Geometry check sheet. Reference: the model listing, model coordinates, mm. Face numbers are marked on the shaded views. A direction names the side the tool comes from. Give positions to 0.01 mm unless a question says otherwise; leave off trailing zeros. Loops run counter-clockwise (first coordinate to the right, second up) from the corner with the lowest first, then second, coordinate; pieces in that order, holes last. Notation, with made-up numbers: (-18.5, 22) -> (18.5, 22) arc R23 ccw to (18.5, 31) -> close; hole circle Ø6 at (32, 75). An arc over 180 degrees is marked (long way). Answer in a Markdown table with one row per item. Add a question column.
```python
from build123d import *

# Parameters (mm, degrees)
SKETCH1_R           = 43.5
BOSS_EXTRUDE1_DEPTH = 11.35
CHAMFER1_SIZE       = 2
SKETCH2_R           = 10.5


with BuildPart() as part:
    # Sketch1 → Boss-Extrude1 (new, symmetric)
    with BuildSketch(Plane.XY):
        Circle(SKETCH1_R)
        with BuildLine():
            Line((-5, 18.142135624), (5, 18.142135624))
            Line((5, 18.142135624), (5, 14.142135624))
            ThreePointArc((5, 14.142135624), (0, -15), (-5, 14.142135624))
            Line((-5, 14.142135624), (-5, 18.142135624))
        make_face(mode=Mode.SUBTRACT)
    extrude(amount=BOSS_EXTRUDE1_DEPTH, both=True)

    # Chamfer1
    chamfer1_edges = [part.edges().sort_by_distance(p)[0] for p in [
        (-43.5, 0, -11.35),
        (-43.5, 0, 11.35),
    ]]
    chamfer(chamfer1_edges, length=CHAMFER1_SIZE)

    # Sketch2 → Cut-Revolve1 (revolve, cut)
    with BuildSketch(Plane(origin=(0, 0, 0), x_dir=(0, 0, -1), z_dir=(1, 0, 0)), mode=Mode.PRIVATE) as cut_revolve1_sk:
        with Locations((0, -52)):
            Circle(SKETCH2_R)
    revolve(cut_revolve1_sk.sketch.rotate(Axis((0, 0, -83.533331893), (0, 0, 1)), 270), axis=Axis((0, 0, -83.533331893), (0, 0, 1)), mode=Mode.SUBTRACT)


solid = part.part
```
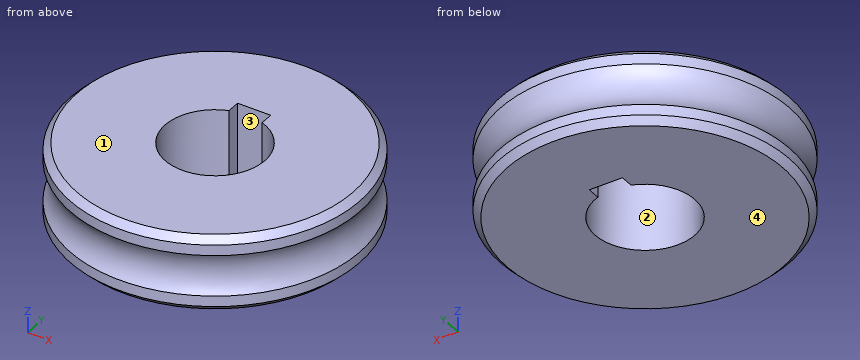
1. Sectioned sample at B-B (x = 0). Enter the section's corners in (y, z), plus the area to 3 significant figures.
2. Sectioned sample at C-C (z = 3.5). Enter the section's corners in (x, y).
3. Gauge pin test, flat ends, axial feed: pin 1 Ø3 at (y, z) = (16.5, 1.5) entering from -X; pin 2 Ø6 at (y, z) = (27.5, -1.5) entering from -X; pin 3 Ø12 at (x, z) = (7.5, -5.5) entering from -Y. Record the tip position at first contact, or that the pin passes through.
4. Sectioned sample at D-D (z = -1.75). Enter the section's corners in (x, y).
5. Release check for a two-part mould opening along Y. For the marked faces 1 and 2 record: released by +Y, released by -Y, zero draft, split by the parting line, or undercut.
6. Access from +Z, -Z, +X, -X, +Y, -Y to the whole of each face (thin tool, end or side, straight path). Record for the marked faces 3 and 4.
7. Material ranges on L1, parallel to Y at x = 0, z = 6.25; L2, parallel to Z at x = -31, y = 29.5; L3, parallel to X at y = 13, z = 7.5, recorded low to high. Write a range as from..to.
8. Sectioned sample at A-A (y = 0). Enter the section's corners in (x, z).
Response:
| question | item | result |
|---|---|---|
| 1 | outline | (-43.5, -9.35) -> (-41.5, -11.35) -> (-15, -11.35) -> (-15, 11.35) -> (-41.5, 11.35) -> (-43.5, 9.35) -> (-43.5, 6.16) arc R10.5 cw to (-43.5, -6.16) -> close; (18.14, -11.35) -> (41.5, -11.35) -> (43.5, -9.35) -> (43.5, -6.16) arc R10.5 cw to (43.5, 6.16) -> (43.5, 9.35) -> (41.5, 11.35) -> (18.14, 11.35) -> close |
| 1 | area | 1,180 mm2 |
| 2 | outline | circle Ø84.2 at (0, 0); hole (-5, 14.14) arc R15 ccw (long way) to (5, 14.14) -> (5, 18.14) -> (-5, 18.14) -> close |
| 3 | pin 1 | stops at x = -38.88 |
| 3 | pin 2 | stops at x = -33.75 |
| 3 | pin 3 | stops at y = -43.47 |
| 4 | outline | circle Ø83.29 at (0, 0); hole (-5, 14.14) arc R15 ccw (long way) to (5, 14.14) -> (5, 18.14) -> (-5, 18.14) -> close |
| 5 | face 1 | zero draft |
| 5 | face 2 | undercut |
| 6 | face 3 | +Z, -Z |
| 6 | face 4 | -Z, +X, -X, +Y, -Y |
| 7 | L1 | y = -43.5..-15, 18.14..43.5 |
| 7 | L2 | z = -10.06..-5.05, 5.05..10.06 |
| 7 | L3 | x = -41.51..-7.48, 7.48..41.51 |
| 8 | outline | (-43.5, -9.35) -> (-41.5, -11.35) -> (-15, -11.35) -> (-15, 11.35) -> (-41.5, 11.35) -> (-43.5, 9.35) -> (-43.5, 6.16) arc R10.5 cw to (-43.5, -6.16) -> close; (15, -11.35) -> (41.5, -11.35) -> (43.5, -9.35) -> (43.5, -6.16) arc R10.5 cw to (43.5, 6.16) -> (43.5, 9.35) -> (41.5, 11.35) -> (15, 11.35) -> close |
